```python
from build123d import *

# Parameters (mm, degrees)
SKETCH1_R           = 0.75
BOSS_EXTRUDE1_DEPTH = 19.5
SKETCH2_R           = 1.5
BOSS_EXTRUDE2_DEPTH = 19.5
SKETCH4_R           = 1.5
BOSS_EXTRUDE3_DEPTH = 4


with BuildPart() as part:
    # Sketch1 → Boss-Extrude1 (new body)
    with BuildSketch(Plane.XY):
        Circle(SKETCH1_R)
    extrude(amount=BOSS_EXTRUDE1_DEPTH)

    # Sketch2 → Boss-Extrude2 (add)
    with BuildSketch(Plane.XY.offset(19.5)):
        Circle(SKETCH2_R)
    extrude(amount=-BOSS_EXTRUDE2_DEPTH)

    # Sketch4 → Boss-Extrude3 (add)
    with BuildSketch(Plane(origin=(0, 0, 0), x_dir=(-1, 0, 0), z_dir=(0, 0, -1))):
        with Locations(Location((0, 0, 0), (0, 0, 180))):
            Circle(SKETCH4_R)
    extrude(amount=BOSS_EXTRUDE3_DEPTH)


solid = part.part
```
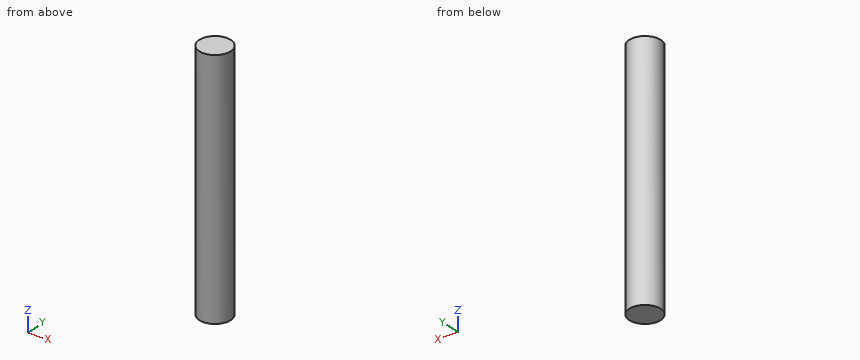
The listing builds one solid part. Answer for the finished solid, in the listing's coordinates (mm). Round coordinates to 2 decimals unless told otherwise and drop trailing zeros. Loops run counter-clockwise (first coordinate to the right, second up) from the corner with the lowest first, then second, coordinate; pieces in that order, holes last. Notation, with made-up numbers: (9.5, 89.25) - (25.5, 89.25) arc R16 ccw to (25.5, 96.25) - close; hole circle Ø5 at (15.5, 5). An arc over 180 degrees is marked (long way). Return JSON: item names as keys, results as strings. Group by question number.
1. The part is cut by section B-B on y = -0.45. Determine the outline of the cut face in (x, z), then the cut area to 3 significant figures.
2. Consider probe 1 along Y at (x, z) = (-1, 8.5); probe 2 along X at (y, z) = (1.2, 6); probe 3 along X at (y, z) = (0.4, -0.25). Determine where each line is inside the solid, lowest interval first.
3. The part is cut by section A-A on z = 8.75. Determine the outline of the cut face in (x, y).
4. The part is cut by section C-C on x = 0.35. Determine the outline of the cut face in (y, z).
Resolved:
{
 "1": {"outline": "(-1.43, -4) - (1.43, -4) - (1.43, 19.5) - (-1.43, 19.5) - close", "area": "67.3 mm²"},
 "2": {"probe 1": "y = -1.12 to 1.12", "probe 2": "x = -0.9 to 0.9", "probe 3": "x = -1.45 to 1.45"},
 "3": {"outline": "circle Ø3 at (0, 0)"},
 "4": {"outline": "(-1.46, -4) - (1.46, -4) - (1.46, 19.5) - (-1.46, 19.5) - close"}
}
